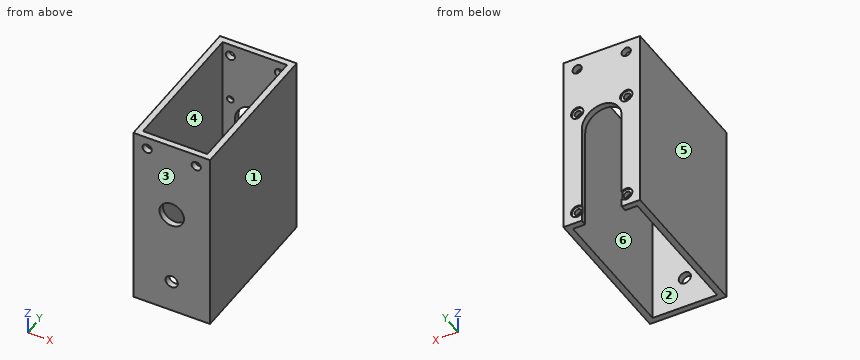
Autodesk Inventor part; units mm, degrees
ref_plane "YZ Plane" through (0, 0, 0) normal (1, 0, 0) x (0, 1, 0)
ref_plane "XZ Plane" through (0, 0, 0) normal (0, 1, 0) x (-1, 0, 0)
ref_plane "XY Plane" through (0, 0, 0) normal (0, 0, 1) x (1, 0, 0)
sketch "スケッチ1" plane through (0, 0, 0) normal (0, 0, 1) x (1, 0, 0)
  line L0 (-12.5, 25) -> (12.5, 25)
  line L1 (12.5, 25) -> (12.5, -25)
  line L2 (12.5, -25) -> (-12.5, -25)
  line L3 (-12.5, -25) -> (-12.5, 25)
  line L4 (-10.5, 23) -> (10.5, 23)
  line L5 (10.5, 23) -> (10.5, -23)
  line L6 (10.5, -23) -> (-10.5, -23)
  line L7 (-10.5, -23) -> (-10.5, 23)
  point P0 (0, 0)
  dimension "d0" = 25
  dimension "d1" = 50
  dimension "d2" = 46
  dimension "d3" = 21
  dimension "d4" = 25
  dimension "d5" = 23
  dimension "d6" = 10.5
  dimension "d7" = 12.5
extrude "押し出し1" add sketch "スケッチ1" along normal blind 60
sketch "スケッチ2" plane through (-12.5, 25, 0) normal (0, 1, 0) x (1, 0, 0)
  line L0 (0, 0) -> (25, 0)
  line L1 (0, 0) -> (0, -60)
  arc A0 (6, -33.5) -> (19, -33.5) centre (12.5, -33.5) ccw
  line L2 (6, -33.5) -> (6, 0)
  line L3 (19, -33.5) -> (19, 0)
  point P0 (12.5, 0)
  dimension "d10" = 13
  dimension "d11" = 33.5
  dimension "d12" = 12.5
extrude "押し出し2" cut sketch "スケッチ2" against normal blind 2
sketch "スケッチ3" plane through (-12.5, 25, 60) normal (0, 1, 0) x (1, 0, 0)
  arc A0 (6, 26.5) -> (19, 26.5) centre (12.5, 26.5) ccw
  circle A1 centre (4.5, 20) radius 1.1
  circle A2 centre (4.5, 56) radius 1.1
  circle A3 centre (20.5, 56) radius 1.1
  circle A4 centre (20.5, 20) radius 1.1
  point P0 (12.5, 60)
  dimension "d15" = 6.5
  dimension "d16" = 6.5
  dimension "d17" = 2.2
  dimension "d18" = 8
  dimension "d19" = 8
  dimension "d20" = 8
  dimension "d21" = 8
  dimension "d22" = 29.5
  dimension "d23" = 29.5
hole "穴1" at (-8, 25, 4) at (8, 25, 4) at (8, 25, 40) at (-8, 25, 40) direction (0, -1, 0) diameter 2.2 depth 2 tip angle 118 counterbore diameter 4 counterbore depth 0.5
sketch "スケッチ4" plane through (-12.5, -25, 0) normal (0, -1, 0) x (1, 0, 0)
  line L0 (25, 0) -> (0, 0)
  line L1 (25, 0) -> (25, 60)
  circle A0 centre (12.5, 10.5) radius 2
  point P0 (12.5, 0)
  dimension "d31" = 4
  dimension "d32" = 12.5
  dimension "d33" = 10.5
hole "穴2" at (0, -25, 10.5) direction (0, 1, 0) diameter 4 end through all
sketch "スケッチ5" plane through (-12.5, 25, 60) normal (0, 1, 0) x (1, 0, 0)
  line L0 (0, 0) -> (25, 0)
  arc A0 (6, 26.5) -> (19, 26.5) centre (12.5, 26.5) ccw
  circle A1 centre (20.5, 4) radius 1.5
  circle A2 centre (4.5, 4) radius 1.5
  point P0 (12.5, 60)
  dimension "d43" = 4
  dimension "d44" = 4
  dimension "d46" = 8
  dimension "d47" = 8
  dimension "d57" = 3
hole "穴4" at (-8, 25, 56) at (8, 25, 56) direction (0, -1, 0) diameter 3 end through all
thread "ねじ1"
thread "ねじ2"
thread "ねじ3"
thread "ねじ4"
sketch "スケッチ7" plane through (-12.5, -25, 0) normal (0, -1, 0) x (1, 0, 0)
  line L0 (25, 60) -> (0, 60)
  line L1 (25, 0) -> (25, 60)
  circle A0 centre (12.5, 35) radius 4
  point P0 (12.5, 0)
  dimension "d78" = 25
  dimension "d79" = 8
  dimension "d80" = 12.5
hole "穴5" at (0, -25, 35) direction (0, 1, 0) diameter 8 end through all
properties part number "07" material "アルミニウム 6061"
CAD build for the part. Positions are in the model's coordinates, mm. Face numbers are marked on the shaded views. A direction names the side the tool comes from. Give positions to 0.01 mm unless a question says otherwise; leave off trailing zeros. Loops run counter-clockwise (first coordinate to the right, second up) from the corner with the lowest first, then second, coordinate; pieces in that order, holes last. Notation, with made-up numbers: (35.5, 62) -> (47.5, 62) arc R14 ccw to (47.5, 89) -> close; hole circle Ø8 at (70.25, 51.5). An arc over 180 degrees is marked (long way). Use a Markdown table: item, result.
1. Flat gauge pins, fed straight in: pin 1 (2 mm diameter, centred on x = 8, z = 40, fed in from +Y); pin 2 (2.5 mm diameter, centred on x = -8, z = 40, fed in from +Y). Where does each tip first touch, or does it go through?
Check result:
| item | result |
|---|---|
| pin 1 | stops at y = -23 |
| pin 2 | stops at y = 24.5 |
2. Slice it at B-B (y = -3.5). List the corners of the cut face in (x, z), plus the area to 3 significant figures.
Check result:
| item | result |
|---|---|
| outline | (-12.5, 0) -> (-10.5, 0) -> (-10.5, 60) -> (-12.5, 60) -> close; (10.5, 0) -> (12.5, 0) -> (12.5, 60) -> (10.5, 60) -> close |
| area | 240 mm^2 |
3. Mould opens along Y. For the marked faces 1, 2, 3 and 4 say: pulls with the +Y half, pulls with the -Y half, needs draft (parallel to the pull), parting line crosses it, or undercut.
Check result:
| item | result |
|---|---|
| face 1 | needs draft |
| face 2 | undercut |
| face 3 | pulls with the -Y half |
| face 4 | undercut |
4. Slice it at D-D (z = 56). List the corners of the cut face in (x, y).
Check result:
| item | result |
|---|---|
| outline | (-12.5, -25) -> (-9.5, -25) -> (-9.5, -23) -> (-10.5, -23) -> (-10.5, 23) -> (-9.5, 23) -> (-9.5, 25) -> (-12.5, 25) -> close; (-6.5, -25) -> (6.5, -25) -> (6.5, -23) -> (-6.5, -23) -> close; (-6.5, 23) -> (6.5, 23) -> (6.5, 25) -> (-6.5, 25) -> close; (9.5, -25) -> (12.5, -25) -> (12.5, 25) -> (9.5, 25) -> (9.5, 23) -> (10.5, 23) -> (10.5, -23) -> (9.5, -23) -> close |
5. Wall check: L1, parallel to Z at x = -8, y = 24.1; L2, parallel to X at y = 24.2, z = 56; L3, parallel to Z at x = 0, y = -24.25. Give the ranges that are in metal, low to high. Write a range as [from, to].
Check result:
| item | result |
|---|---|
| L1 | z = [0, 2.9], [5.1, 38.9], [41.1, 54.5], [57.5, 60] |
| L2 | x = [-12.5, -9.5], [-6.5, 6.5], [9.5, 12.5] |
| L3 | z = [0, 8.5], [12.5, 31], [39, 60] |
6. Slice it at A-A (z = 4). List the corners of the cut face in (x, y), plus the area to 3 significant figures.
Check result:
| item | result |
|---|---|
| outline | (-12.5, -25) -> (12.5, -25) -> (12.5, 25) -> (10, 25) -> (10, 24.5) -> (9.1, 24.5) -> (9.1, 23) -> (10.5, 23) -> (10.5, -23) -> (-10.5, -23) -> (-10.5, 23) -> (-9.1, 23) -> (-9.1, 24.5) -> (-10, 24.5) -> (-10, 25) -> (-12.5, 25) -> close; (-6.9, 23) -> (-6.5, 23) -> (-6.5, 24.5) -> (-6.9, 24.5) -> close; (6.5, 23) -> (6.9, 23) -> (6.9, 24.5) -> (6.5, 24.5) -> close |
| area | 248 mm^2 |
7. Which spindle directions (+Z, -Z, +X, -X, +Y, -Y) get a long thin tool onto all of the face, cutting with end or side? Do the marked faces 5 and 6. Say none if no direction does.
Check result:
| item | result |
|---|---|
| face 5 | +Z, -Z, -X, +Y, -Y |
| face 6 | +Z, -Z |
8. Slice it at C-C (x = 0). List the corners of the cut face in (y, z), plus the area to 3 significant figures.
Check result:
| item | result |
|---|---|
| outline | (-25, 0) -> (-23, 0) -> (-23, 8.5) -> (-25, 8.5) -> close; (-25, 12.5) -> (-23, 12.5) -> (-23, 31) -> (-25, 31) -> close; (-25, 39) -> (-23, 39) -> (-23, 60) -> (-25, 60) -> close; (23, 40) -> (25, 40) -> (25, 60) -> (23, 60) -> close |
| area | 136 mm^2 |
